from build123d import *

# Parameters (mm, degrees)
SKETCH_1_W          = 20
SKETCH_1_H          = 20
SKETCH_1_W_2        = 10
SKETCH_1_H_2        = 10
EXTRUDE_1_DEPTH     = 20
SKETCH_2_W          = 20
SKETCH_2_H          = 3
EXTRUDE_2_DEPTH     = 5
EXTRUDE_3_DEPTH     = 20
SKETCH_4_W          = 8
SKETCH_4_H          = 1.5
CUT_EXTRUDE_1_DEPTH = 20


with BuildPart() as part:
    # 草图1 → 凸台-拉伸1 (new body)
    with BuildSketch(Plane.XY):
        with Locations((5, 5)):
            Rectangle(SKETCH_1_W, SKETCH_1_H)
        with Locations((5, 5)):
            Rectangle(SKETCH_1_W_2, SKETCH_1_H_2, mode=Mode.SUBTRACT)
    extrude(amount=EXTRUDE_1_DEPTH)

    # 草图2 → 凸台-拉伸2 (add)
    with BuildSketch(Plane(origin=(0, 0, 0), x_dir=(-1, 0, 0), z_dir=(0, 0, -1))):
        with Locations((-5, 11.5)):
            Rectangle(SKETCH_2_W, SKETCH_2_H)
        with Locations((-5, -1.5)):
            Rectangle(SKETCH_2_W, SKETCH_2_H)
    extrude(amount=EXTRUDE_2_DEPTH)

    # 草图3 → 凸台-拉伸3 (add)
    with BuildSketch(Plane.ZY.offset(5)):
        Polygon((-5, 10), (-5, 9.5), (-8, 10), (-8, 13), (-5, 13), align=None)
        Polygon((-5, 0), (-5, 0.5), (-8, 0), (-8, -3), (-5, -3), align=None)
    extrude(amount=-EXTRUDE_3_DEPTH)

    # 草图4 → 切除-拉伸1 (cut)
    with BuildSketch(Plane.ZY.offset(5)):
        with Locations((-4, 12.25)):
            Rectangle(SKETCH_4_W, SKETCH_4_H)
        with Locations((-4, -2.25)):
            Rectangle(SKETCH_4_W, SKETCH_4_H)
    extrude(amount=-CUT_EXTRUDE_1_DEPTH, mode=Mode.SUBTRACT)


solid = part.part
Part model, mm, in its own coordinate system. A direction names the side the tool comes from. Give positions to 0.01 mm unless a question says otherwise; leave off trailing zeros. Loops run counter-clockwise (first coordinate to the right, second up) from the corner with the lowest first, then second, coordinate; pieces in that order, holes last.
(1) Band-saw the part on D-D (z = -2.75). Write the cut outline in (x, y), and give its area (3 significant figures).
Return value:
outline: (-5, -1.5) - (15, -1.5) - (15, 0) - (-5, 0) - close; (-5, 10) - (15, 10) - (15, 11.5) - (-5, 11.5) - close
area: 60.0 mm2
(2) Band-saw the part on B-B (z = 15.25). Write the cut outline in (x, y).
Return value:
outline: (-5, -5) - (15, -5) - (15, 15) - (-5, 15) - close; hole (0, 0) - (10, 0) - (10, 10) - (0, 10) - close
(3) 3-axis set-ups, long thin cutter, end or side, ignore diameter. For faces 1 (the flat face through (5, 10, 5)), 2 (the flat face through (5, -3, 0)), 3 (the flat face through (4.86, 0.253, -6.479)): which of +Z, -Z, +X, -X, +Y, -Y reach the whole face in a straight line?
Return value:
face 1: none
face 2: -Z, +X, -X, -Y
face 3: -Z, +X, -X
(4) Drill centre lines: line 1 along X through (y, z) = (3, 3); line 2 along Y through (x, z) = (6.5, -1). Where is each one in solid material? Low to high.
Return value:
line 1: x = -5 to 0, 10 to 15
line 2: y = -1.5 to 0, 10 to 11.5
(5) Pull direction X, two halves, no side cores. Call faces 4 (the flat face through (5, 11, -8)), 5 (the flat face through (5, 0, 5)), 6 (the flat face through (-5, 5, 12)): pulls with the +X half, pulls with the -X half, needs draft (parallel to the pull), parting line crosses it, or undercut.
Return value:
face 4: needs draft
face 5: undercut
face 6: pulls with the -X half
(6) Band-saw the part on A-A (x = 2.5). Write the cut outline in (y, z), and give its area (4 significant figures).
Return value:
outline: (-5, 0) - (-1.5, 0) - (-1.5, -8) - (0, -8) - (0.5, -5) - (0, -5) - (0, 20) - (-5, 20) - close; (9.5, -5) - (10, -8) - (11.5, -8) - (11.5, 0) - (15, 0) - (15, 20) - (10, 20) - (10, -5) - close
area: 225.5 mm2
(7) Band-saw the part on C-C (y = 4.75). Write the cut outline in (x, z), and give its area (3 significant figures).
Return value:
outline: (-5, 0) - (0, 0) - (0, 20) - (-5, 20) - close; (10, 0) - (15, 0) - (15, 20) - (10, 20) - close
area: 200 mm2
(8) Pin check, flat tips, straight feed: pin 1 (6.5 mm diameter, centred on x = 4, z = -3.5, fed in from -Y); pin 2 (2.5 mm diameter, centred on x = 11.5, y = 4, fed in from -Z); pin 3 (4 mm diameter, centred on x = 8, z = -5.5, fed in from +Y). Stop position of each tip, or through.
Return value:
pin 1: stops at y = -1.5
pin 2: stops at z = 0
pin 3: stops at y = 11.5
